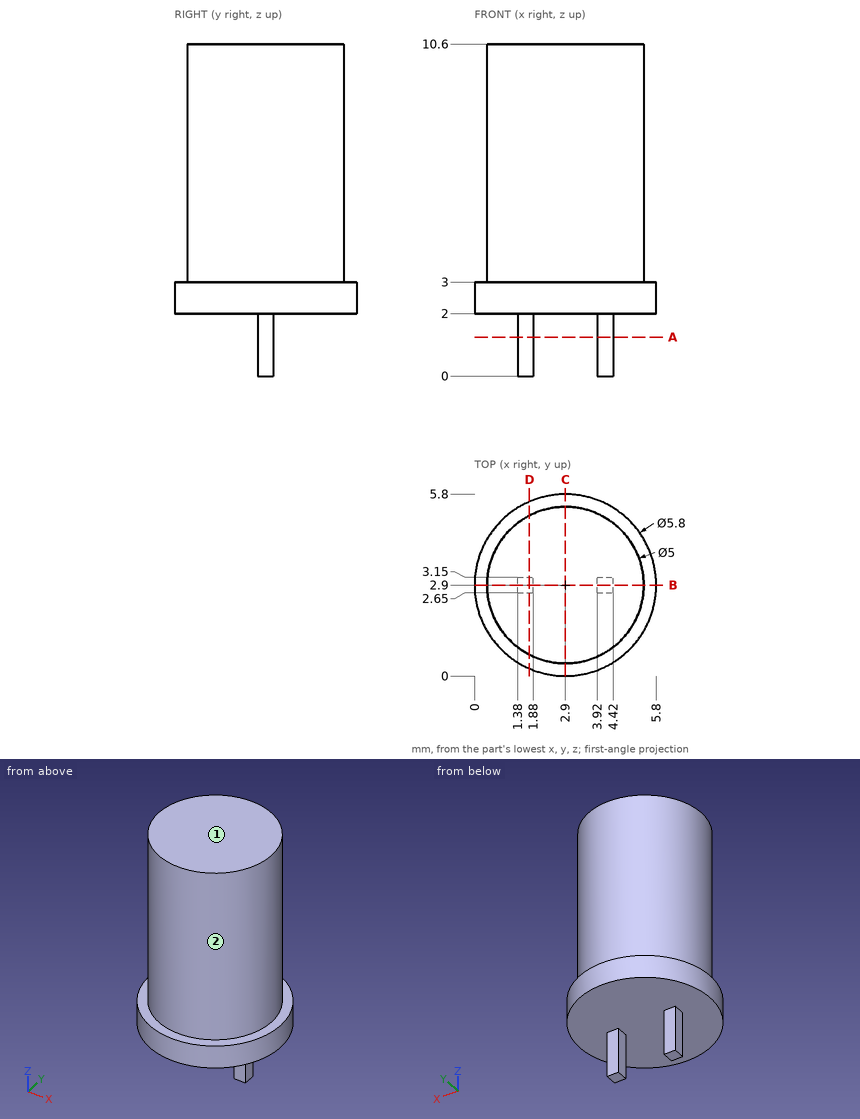
Answer from the drawing. Dimensions are ordinates in mm from the lowest x, y and z of the part. A direction names the side the tool comes from. Round coordinates to 2 decimals unless told otherwise and drop trailing zeros. Write each loop counter-clockwise with the first axis right and the second up, starting at its lowest first coordinate (ties: lowest second). Pieces come first, ordered by that corner, then holes. Notation, with made-up numbers: (-31, -9) -> (3, -9) arc R22 cw to (3, 6) -> close; hole circle Ø10 at (58, 28). An arc over 180 degrees is marked (long way). Write each question's results on one line, items separated by ' | '.
1) The part is cut by section A-A (z = 1.25). Write down the section's boundary in (x, y), and give its area (3 significant figures).
Findings:
outline: (1.38, 2.65) -> (1.88, 2.65) -> (1.88, 3.15) -> (1.38, 3.15) -> close; (3.92, 2.65) -> (4.42, 2.65) -> (4.42, 3.15) -> (3.92, 3.15) -> close | area: 0.500 mm²
2) The part is cut by section B-B (y = 2.9). Write down the section's boundary in (x, z).
Findings:
outline: (0, 2) -> (1.38, 2) -> (1.38, 0) -> (1.88, 0) -> (1.88, 2) -> (3.92, 2) -> (3.92, 0) -> (4.42, 0) -> (4.42, 2) -> (5.8, 2) -> (5.8, 3) -> (5.4, 3) -> (5.4, 10.6) -> (0.4, 10.6) -> (0.4, 3) -> (0, 3) -> close
3) The part is cut by section D-D (x = 1.75). Write down the section's boundary in (y, z).
Findings:
outline: (0.24, 2) -> (2.65, 2) -> (2.65, 0) -> (3.15, 0) -> (3.15, 2) -> (5.56, 2) -> (5.56, 3) -> (5.12, 3) -> (5.12, 10.6) -> (0.68, 10.6) -> (0.68, 3) -> (0.24, 3) -> close
4) Which of the six approach directions +Z, -Z, +X, -X, +Y, -Y give full straight-line access (tool end or side, diameter ignored) to the marked faces 1 and 2?
Findings:
face 1: +Z, +X, -X, +Y, -Y | face 2: +Z
5) The part is cut by section C-C (x = 2.9). Write down the section's boundary in (y, z), and give its area (3 significant figures).
Findings:
outline: (0, 2) -> (5.8, 2) -> (5.8, 3) -> (5.4, 3) -> (5.4, 10.6) -> (0.4, 10.6) -> (0.4, 3) -> (0, 3) -> close | area: 43.8 mm²
6) Consider line 1 along Z through (x, y) = (1.1, 1.2); line 2 along Y through (x, z) = (4.8, 4); line 3 along X through (y, z) = (2.3, 9). Determine where each line is inside the solid, lowest interval first. Write a range as [from, to].
Findings:
line 1: z = [2, 10.6] | line 2: y = [1.28, 4.52] | line 3: x = [0.47, 5.33]
7) Flat-ended cylindrical pins translate along their axes: pin 1 (1.5 mm diameter, centred on x = 2, z = 8, fed in from +Y); pin 2 (0.6 mm diameter, centred on x = 1.5, z = 1.5, fed in from -Y); pin 3 (1 mm diameter, centred on x = 2.5, y = 1, fed in from -Z). Find the tip coordinate at first contact, or state that the pin passes through.
Findings:
pin 1: stops at y = 5.4 | pin 2: stops at y = 2.65 | pin 3: stops at z = 2
